from build123d import *

# Parameters (mm, degrees)
SALIENTE_EXTRUIR1_DEPTH                              = 30
TALADRO_ROSCADO_M4X0_71_D                            = 3.3
TALADRO_ROSCADO_M4X0_71_DEPTH                        = 15
TALADRO_ROSCADO_M4X0_71_TIP                          = 0.991420021
REFRENTADO_PARA_TORNILLO_TAP_N_CON_CABEZ_D           = 5.3
REFRENTADO_PARA_TORNILLO_TAP_N_CON_CABEZ_CBORE_D     = 9
REFRENTADO_PARA_TORNILLO_TAP_N_CON_CABEZ_CBORE_DEPTH = 5
CROQUIS9_R                                           = 2.65
SALIENTE_EXTRUIR2_DEPTH                              = 19
TALADRO_ROSCADO_M5X0_82_D                            = 4.5


with BuildPart() as part:
    # Croquis1 → Saliente-Extruir1 (new body)
    with BuildSketch(Plane.XY):
        with BuildLine():
            Line((-20, -30), (20, -30))
            Line((20, -30), (20, 30))
            Line((20, 30), (1, 30))
            Line((1, 30), (1, 20.968719423))
            ThreePointArc((1, 20.968719423), (0, -11), (-1, 20.968719423))
            Line((-1, 20.968719423), (-1, 30))
            Line((-1, 30), (-20, 30))
            Line((-20, 30), (-20, -30))
        make_face()
    extrude(amount=SALIENTE_EXTRUIR1_DEPTH)

    # Taladro roscado M4x0.71
    with Locations(Plane(origin=(0, -30, 0), x_dir=(-1, 0, 0), z_dir=(0, -1, 0))):
        with Locations((-15, -5), (-15, -25), (15, -5), (15, -25)):
            Hole(TALADRO_ROSCADO_M4X0_71_D / 2, depth=TALADRO_ROSCADO_M4X0_71_DEPTH)
            with Locations((0, 0, -(TALADRO_ROSCADO_M4X0_71_DEPTH + TALADRO_ROSCADO_M4X0_71_TIP / 2))):  # 118° drill point
                Cone(0, TALADRO_ROSCADO_M4X0_71_D / 2, TALADRO_ROSCADO_M4X0_71_TIP, mode=Mode.SUBTRACT)

    # Refrentado para tornillo tapón con cabeza de clavija de M52 (through all)
    with Locations(Plane(origin=(20, 0, 0), x_dir=(0, 0, -1), z_dir=(1, 0, 0))):
        with Locations((-15, 25)):
            CounterBoreHole(REFRENTADO_PARA_TORNILLO_TAP_N_CON_CABEZ_D / 2, REFRENTADO_PARA_TORNILLO_TAP_N_CON_CABEZ_CBORE_D / 2, REFRENTADO_PARA_TORNILLO_TAP_N_CON_CABEZ_CBORE_DEPTH)

    # Croquis9 → Saliente-Extruir2 (add)
    with BuildSketch(Plane.ZY.offset(20)):
        with Locations(Location((15, 25, 0), (0, 0, 180))):
            Circle(CROQUIS9_R)
    extrude(amount=-SALIENTE_EXTRUIR2_DEPTH)

    # Taladro roscado M5x0.82 (through all)
    with Locations(Plane.ZY.offset(20)):
        with Locations((15, 25)):
            Hole(TALADRO_ROSCADO_M5X0_82_D / 2)


solid = part.part
Geometry: final body of the model. Coordinates: model frame, mm. A direction names the side the tool comes from. Give positions to 0.01 mm unless a question says otherwise; leave off trailing zeros. Loops run counter-clockwise (first coordinate to the right, second up) from the corner with the lowest first, then second, coordinate; pieces in that order, holes last. Notation, with made-up numbers: M 10,-20.5 L 15,-20.5 A19 ccw 15,-11.5 Z; hole C 85,78 d6. An arc over 180 degrees is marked long. Put each result on its own line as item: value. Start each with the question number.
1) Pull-direction query (Y, two-part tool) for faces 4 (the cylindrical face through (16.574, -22.395, 4.504)), 5 (the conical face through (15.23, -14.18, 5.17)), 6 (the cylindrical face through (0.689, -10.985, 14.79)); classes: pulls with the +Y half, pulls with the -Y half, needs draft (parallel to the pull), parting line crosses it, or undercut.
2) Access query for faces 1 (the cylindrical face through (-14.11, -22.4, 23.61)), 2 (the cylindrical face through (7.9, 23.99, 17.45)), 3 (the flat face through (-1, 27.4, 14.8)). Directions: +Z, -Z, +X, -X, +Y, -Y. A direction counts if a zero-diameter tool reaches every point of the face in a straight line with its end or side. Return the directions, or none.
3) Cut plane B-B (y = 5). Output: boundary loops of the cut face in (x, z).
4) Cut plane C-C (z = 14). Output: boundary loops of the cut face in (x, y), then the cut area to 3 significant figures.
5) Cut plane D-D (y = 25). Output: boundary loops of the cut face in (x, z).
6) Ray query, line 1 along X through (y, z) = (-18, 25); line 2 along Z through (x, y) = (-15, -22); line 3 along X through (y, z) = (24.5, 4). Return the intervals inside material, ascending.
7) Cut plane A-A (x = 3). Output: boundary loops of the cut face in (y, z), then the cut area to 3 significant figures.
8) Contact query for flat-ended pins moving along their axis: pin 1 (4.5 mm diameter, centred on y = 27, z = 14.5, fed in from -X); pin 2 (3 mm diameter, centred on y = 25, z = 15, fed in from -X); pin 3 (3 mm diameter, centred on x = 15, z = 25, fed in from -Y); pin 4 (2.5 mm diameter, centred on y = 24, z = 14.5, fed in from +X). Output: stop coordinate, or through.
Verdict:
1. face 4: needs draft
1. face 5: pulls with the -Y half
1. face 6: undercut
2. face 1: -Y
2. face 2: +X
2. face 3: +Z, -Z, +Y
3. outline: M -20,0 L -16,0 L -16,30 L -20,30 Z; M 16,0 L 20,0 L 20,30 L 16,30 Z
4. outline: M -20,-30 L 20,-30 L 20,20.61 L 15,20.61 L 15,22.55 L 1,22.55 L 1,20.97 A16 cw long -1,20.97 L -1,22.98 L -20,22.98 Z; M -20,27.02 L -1,27.02 L -1,30 L -20,30 Z; M 1,27.45 L 15,27.45 L 15,29.39 L 20,29.39 L 20,30 L 1,30 Z
4. area: 1,390 mm2
5. outline: M -20,0 L -1,0 L -1,12.75 L -20,12.75 Z; M -20,17.25 L -1,17.25 L -1,30 L -20,30 Z; M 1,0 L 20,0 L 20,10.5 L 15,10.5 L 15,12.35 L 1,12.35 Z; M 1,17.65 L 15,17.65 L 15,19.5 L 20,19.5 L 20,30 L 1,30 Z
6. line 1: -20 to -16.65, -13.35 to 13.35, 16.65 to 20
6. line 2: 0 to 3.35, 6.65 to 23.35, 26.65 to 30
6. line 3: -20 to -1, 1 to 20
7. outline: M -30,0 L -10.72,0 L -10.72,30 L -30,30 Z; M 20.72,0 L 30,0 L 30,30 L 20.72,30 Z; hole C 25,15 d5.3
7. area: 835 mm2
8. pin 1: x = -20
8. pin 2: through
8. pin 3: y = -14.91
8. pin 4: x = -1
